from build123d import *

# Parameters (mm, degrees)
EXTRUDE_DEPTH           = 25
EXTRUDE_PLACEMENT_ANGLE = 90


with BuildPart() as part:
    # Sketch → Extrude (new body)
    with BuildSketch(Plane.XY):
        Polygon((0, 11), (0, 0), (60, 0), (60, 11), (54, 11), (55, 3), (43, 3), (43, 11), align=None)
    extrude(amount=EXTRUDE_DEPTH)


with BuildPart() as part_1:
    # Extrude placement: moved
    add(part.part.rotate(Axis((0, 0, 0), (1, 0, 0)), EXTRUDE_PLACEMENT_ANGLE))


solid = part_1.part
Part model, mm, in its own coordinate system. A direction names the side the tool comes from. Give positions to 0.01 mm unless a question says otherwise; leave off trailing zeros. Loops run counter-clockwise (first coordinate to the right, second up) from the corner with the lowest first, then second, coordinate; pieces in that order, holes last. Notation, with made-up numbers: M -15,22 L 36,22 A12 cw 36,32 Z; hole C 4.5,72.5 d11. An arc over 180 degrees is marked long. Put each result on its own line as item: value. Start each with the question number.
1) Saw through at C-C (z = 9.5). List the corners of the cut face in (x, y), then the cut area to 3 significant figures.
2) 3-axis set-ups, long thin cutter, end or side, ignore diameter. For faces 1 (the flat face through (43, -12, 7)), 2 (the flat face through (30, -25, 6)): which of +Z, -Z, +X, -X, +Y, -Y reach the whole face in a straight line?
3) Probe probe 1 along X at (y, z) = (-14.75, 5.5); probe 2 along X at (y, z) = (-11.25, 8) (3 decimals); probe 3 along Z at (x, y) = (52.5, -20.75). List the from-to ranges inside material, lowest first.
4) Saw through at A-A (z = 5). List the corners of the cut face in (x, y), then the cut area to 3 significant figures.
5) Saw through at D-D (x = 44.5). List the corners of the cut face in (y, z).
6) Saw through at B-B (y = -18.5). List the corners of the cut face in (x, z).
7) Pull direction Z, two halves, no side cores. Call faces 3 (the flat face through (60, -12, 5)), 4 (the flat face through (57, -12, 11)), 5 (the flat face through (30, -12, 0)), 6 (the flat face through (54.493, -12.325, 7.056)): +Z half, -Z half, draft (parallel to the pull), parting line (faces both ways), or undercut.
Numbers:
1. outline: M 0,-25 L 43,-25 L 43,0 L 0,0 Z; M 54.19,-25 L 60,-25 L 60,0 L 54.19,0 Z
1. area: 1,220 mm^2
2. face 1: +Z, +Y, -Y
2. face 2: +Z, -Z, +X, -X, -Y
3. probe 1: 0 to 43, 54.69 to 60
3. probe 2: 0 to 43, 54.375 to 60
3. probe 3: 0 to 3
4. outline: M 0,-25 L 43,-25 L 43,0 L 0,0 Z; M 54.75,-25 L 60,-25 L 60,0 L 54.75,0 Z
4. area: 1,210 mm^2
5. outline: M -25,0 L 0,0 L 0,3 L -25,3 Z
6. outline: M 0,0 L 60,0 L 60,11 L 54,11 L 55,3 L 43,3 L 43,11 L 0,11 Z
7. face 3: draft
7. face 4: +Z half
7. face 5: -Z half
7. face 6: undercut
